Work out the finished part from the listing and answer in its coordinate system (mm). Face numbers are marked on the shaded views. A direction names the side the tool comes from. Give positions to 0.01 mm unless a question says otherwise; leave off trailing zeros. Loops run counter-clockwise (first coordinate to the right, second up) from the corner with the lowest first, then second, coordinate; pieces in that order, holes last. Notation, with made-up numbers: M 2.5,-1 L 40.5,-1 A21 cw 40.5,38 Z; hole C 42,19.25 d5. An arc over 180 degrees is marked long. Answer as a JSON object with one key per item and string values. Group by question number.
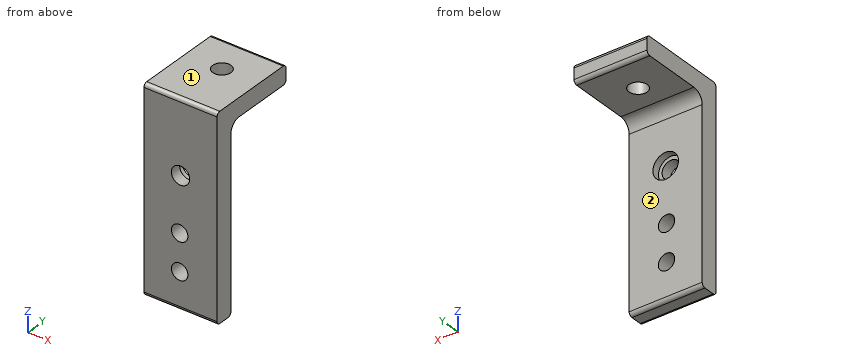
```python
from build123d import *

# Parameters (mm, degrees)
EXTRUDE_1_DEPTH     = 20
FILLET_1_R          = 3
FILLET_2_R          = 1
SKETCH_2_R          = 2.5
CUT_EXTRUDE_1_DEPTH = 20
SKETCH_3_R          = 2.25
SKETCH_3_R_2        = 2.5
CUT_EXTRUDE_2_DEPTH = 20
SKETCH_5_R          = 3.5
CUT_EXTRUDE_3_DEPTH = 2


with BuildPart() as part:
    # 草图1 → 凸台-拉伸1 (new body)
    with BuildSketch(Plane(origin=(0, 0, 0), x_dir=(0, 0, -1), z_dir=(1, 0, 0))):
        Polygon((0, 0), (55, 0), (55, 5), (5, 5), (5, 25), (0, 25), align=None)
    extrude(amount=EXTRUDE_1_DEPTH)

    # 圆角1
    fillet_1_edges = [part.edges().sort_by_distance(p)[0] for p in [
        (10, 5, -5),
    ]]
    fillet(fillet_1_edges, radius=FILLET_1_R)

    # 圆角2
    fillet_2_edges = [part.edges().sort_by_distance(p)[0] for p in [
        (10, 25, 0),
        (10, 25, -5),
        (10, 5, -55),
        (10, 0, -55),
        (10, 0, 0),
    ]]
    fillet(fillet_2_edges, radius=FILLET_2_R)

    # 草图2 → 切除-拉伸1 (cut)
    with BuildSketch(Plane(origin=(0, 0, -5), x_dir=(-1, 0, 0), z_dir=(0, 0, -1))):
        with Locations(Location((-10, 15, 0), (0, 0, 90))):
            Circle(SKETCH_2_R)
    extrude(amount=-CUT_EXTRUDE_1_DEPTH, mode=Mode.SUBTRACT)

    # 草图3 → 切除-拉伸2 (cut)
    with BuildSketch(Plane(origin=(0, 5, 0), x_dir=(1, 0, 0), z_dir=(0, 1, 0))):
        with Locations(Location((9.767852346, 45, 0), (0, 0, 270))):
            Circle(SKETCH_3_R)
        with Locations(Location((9.767852346, 35, 0), (0, 0, 270))):
            Circle(SKETCH_3_R)
        with Locations(Location((10, 20.001796525, 0), (0, 0, 270))):
            Circle(SKETCH_3_R_2)
    extrude(amount=-CUT_EXTRUDE_2_DEPTH, mode=Mode.SUBTRACT)

    # 草图5 → 切除-拉伸3 (cut)
    with BuildSketch(Plane(origin=(0, 5, 0), x_dir=(1, 0, 0), z_dir=(0, 1, 0))):
        with Locations(Location((10, 20.001796525, 0), (0, 0, 270))):
            Circle(SKETCH_5_R)
    extrude(amount=-CUT_EXTRUDE_3_DEPTH, mode=Mode.SUBTRACT)


solid = part.part
```
Item 1: A cutting plane is placed at A-A (y = 15). Determine the outline of the cut face in (x, z).
Item 2: A tool of negligible diameter and unlimited length cuts with its end or side. For the marked faces 1 and 2, from which of +Z, -Z, +X, -X, +Y, -Y can it reach the whole face along a straight path? Write none if from no direction.
Item 3: Given pin 1 Ø8 at (x, y) = (11.5, 17) entering from -Z; pin 2 Ø11 at (x, z) = (10, -20) entering from +Y; pin 3 Ø6.5 at (x, z) = (10, -20) entering from +Y, each flat-ended and moving along its own axis, determine where each tip first touches the part or whether it passes through.
Item 4: Find the intervals of material crossed by probe 1 along X at (y, z) = (2.15, -35); probe 2 along Y at (x, z) = (14.75, -47); probe 3 along Z at (x, y) = (4.5, 23), in increasing order. Write a range as [from, to].
Item 5: A cutting plane is placed at C-C (x = 17.75). Determine the outline of the cut face in (y, z).
Item 6: A cutting plane is placed at D-D (z = -32). Determine the outline of the cut face in (x, y), and give its area (3 significant figures).
Item 7: A cutting plane is placed at B-B (z = -45). Determine the outline of the cut face in (x, y), and give its area (3 significant figures).
The answers:
{
 "1": {"outline": "M 0,-5 L 7.5,-5 L 7.5,0 L 0,0 Z; M 12.5,-5 L 20,-5 L 20,0 L 12.5,0 Z"},
 "2": {"face 1": "+Z, +X, -X, +Y, -Y", "face 2": "-Z, +X, -X, +Y"},
 "3": {"pin 1": "stops at z = -5", "pin 2": "stops at y = 5", "pin 3": "stops at y = 3"},
 "4": {"probe 1": "x = [0, 7.52], [12.02, 20]", "probe 2": "y = [0, 5]", "probe 3": "z = [-5, 0]"},
 "5": {"outline": "M 0,-54 A1 ccw 1,-55 L 4,-55 A1 ccw 5,-54 L 5,-8 A3 cw 8,-5 L 24,-5 A1 ccw 25,-4 L 25,-1 A1 ccw 24,0 L 1,0 A1 ccw 0,-1 Z"},
 "6": {"outline": "M 0,0 L 20,0 L 20,5 L 0,5 Z", "area": "100 mm^2"},
 "7": {"outline": "M 0,0 L 7.52,0 L 7.52,5 L 0,5 Z; M 12.02,0 L 20,0 L 20,5 L 12.02,5 Z", "area": "77.5 mm^2"}
}
